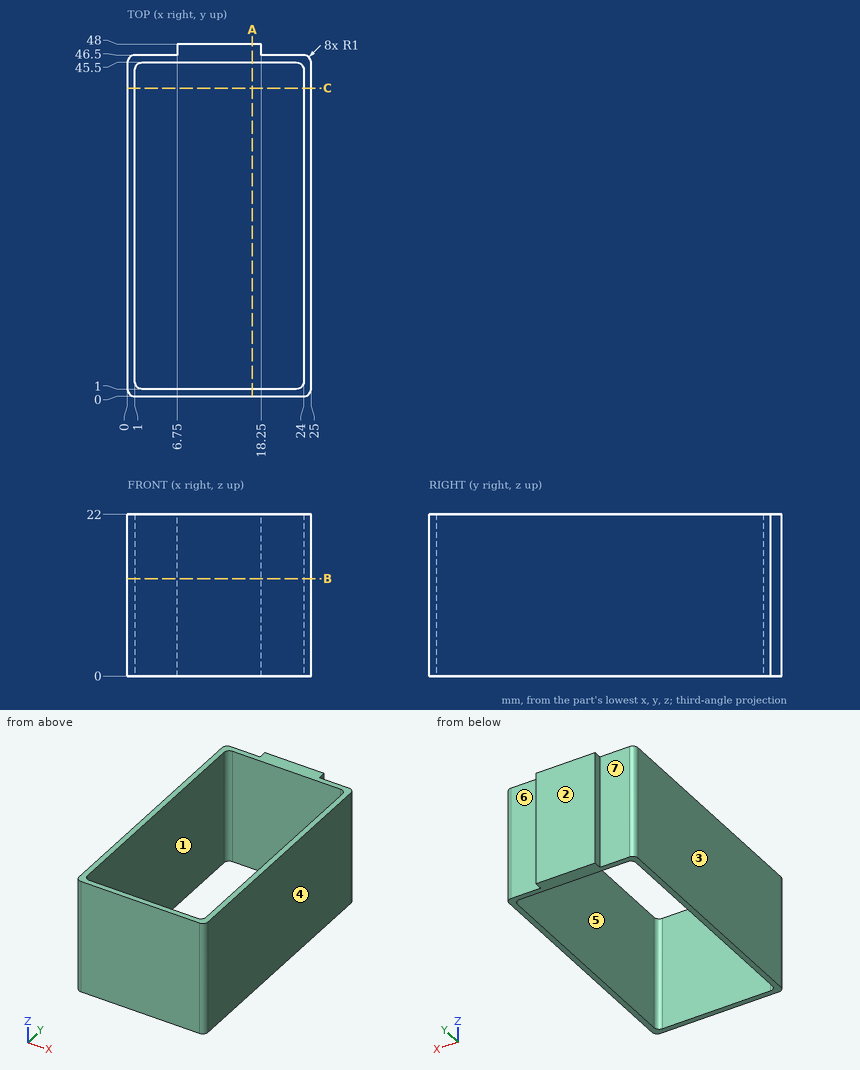
The drawing under review shows one solid part. Ordinate dimensions are in mm from its lowest x, y, z. A direction names the side the tool comes from. Coordinates: 2 decimals unless noted, no trailing zeros. Order: outer loops, then holes, each group sorted by start corner. A loop starts at its lowest first (then second) coordinate and runs counter-clockwise, first axis right, second up. Notation, with made-up numbers: (-36, 3) -> (-7, 3) arc R18 cw to (-7, 18) -> close; hole circle Ø7 at (-33, 47). An arc over 180 degrees is marked (long way). Return JSON: item names as keys, results as strings.
1. For line 1 (Y direction, x = 14.25, z = 8.25); line 2 (X direction, y = 35, z = 16.5); line 3 (Y direction, x = 4.25, z = 1.5), list the stretches that pass through material, from the lowest coordinate up. Write a range as from..to.
Answer block:
{"line 1": "0..1, 45.5..48", "line 2": "0..1, 24..25", "line 3": "0..1, 45.5..46.5"}
2. We need section A-A on x = 17. Write out the cut boundary in (y, z).
Answer block:
{"outline": "(0, 0) -> (1, 0) -> (1, 22) -> (0, 22) -> close; (45.5, 0) -> (48, 0) -> (48, 22) -> (45.5, 22) -> close"}
3. We need section C-C on y = 42. Write out the cut boundary in (x, z), and give its area (3 significant figures).
Answer block:
{"outline": "(0, 0) -> (1, 0) -> (1, 22) -> (0, 22) -> close; (24, 0) -> (25, 0) -> (25, 22) -> (24, 22) -> close", "area": "44.0 mm²"}
4. Machinability: for the marked faces 4, 5, 6 and 7, which of the approach directions +Z, -Z, +X, -X, +Y, -Y give a long, thin tool a straight path to every point of the face, cutting with its end or side? Answer none if there is none.
Answer block:
{"face 4": "+Z, -Z, +X, +Y, -Y", "face 5": "+Z, -Z", "face 6": "+Z, -Z, +X, +Y", "face 7": "+Z, -Z, -X, +Y"}
5. The part is to be moulded in two halves that separate along X. For the marked faces 1, 2 and 3, say which applies: +X half, -X half, draft (parallel to the pull), parting line (faces both ways), or undercut.
Answer block:
{"face 1": "undercut", "face 2": "draft", "face 3": "-X half"}
6. We need section B-B on z = 13.25. Write out the cut boundary in (x, y).
Answer block:
{"outline": "(0, 1) arc R1 ccw to (1, 0) -> (24, 0) arc R1 ccw to (25, 1) -> (25, 45.5) arc R1 ccw to (24, 46.5) -> (18.25, 46.5) -> (18.25, 48) -> (6.75, 48) -> (6.75, 46.5) -> (1, 46.5) arc R1 ccw to (0, 45.5) -> close; hole (1, 2) arc R1 ccw to (2, 1) -> (23, 1) arc R1 ccw to (24, 2) -> (24, 44.5) arc R1 ccw to (23, 45.5) -> (2, 45.5) arc R1 ccw to (1, 44.5) -> close"}
7. For pin 1 Ø4 at (x, y) = (9, 42.5) entering from -Z; pin 2 Ø6.5 at (x, z) = (3, 11) entering from +Y; pin 3 Ø1.2 at (y, z) = (47.5, 7.5) entering from +X; pin 4 Ø0.8 at (y, z) = (47, 15.5) entering from -X, all flat-tipped, find the tip position at first contact; note any pin that passes through.
Answer block:
{"pin 1": "through", "pin 2": "y = 46.5", "pin 3": "x = 18.25", "pin 4": "x = 6.75"}
